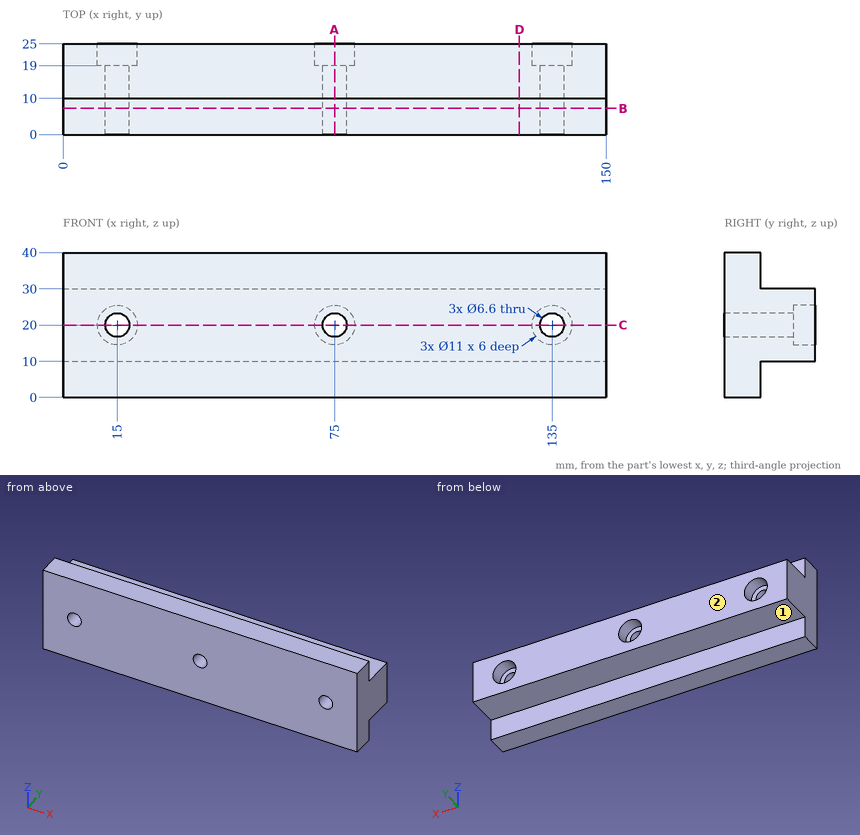
The drawing under review shows one solid part. Ordinate dimensions are in mm from its lowest x, y, z. A direction names the side the tool comes from. Round coordinates to 2 decimals unless told otherwise and drop trailing zeros. Loops run counter-clockwise (first coordinate to the right, second up) from the corner with the lowest first, then second, coordinate; pieces in that order, holes last.
Item 1: For the marked faces 1 and 2, list the 3-axis set-ups (+Z, -Z, +X, -X, +Y, -Y) from which the entire face can be reached by the end or side of a thin tool; tool diameter is ignored.
Determined:
face 1: -Z, +X, -X, +Y
face 2: +Z, -Z, +X, -X, +Y
Item 2: Take a section at A-A (x = 75). Write out the cut boundary in (y, z), then the cut area to 3 significant figures.
Determined:
outline: (0, 0) - (10, 0) - (10, 10) - (25, 10) - (25, 14.5) - (19, 14.5) - (19, 16.7) - (0, 16.7) - close; (0, 23.3) - (19, 23.3) - (19, 25.5) - (25, 25.5) - (25, 30) - (10, 30) - (10, 40) - (0, 40) - close
area: 509 mm2
Item 3: Take a section at D-D (x = 126). Write out the cut boundary in (y, z), then the cut area to 3 significant figures.
Determined:
outline: (0, 0) - (10, 0) - (10, 10) - (25, 10) - (25, 30) - (10, 30) - (10, 40) - (0, 40) - close
area: 700 mm2
Item 4: Take a section at B-B (y = 7.25). Write out the cut boundary in (x, z).
Determined:
outline: (0, 0) - (150, 0) - (150, 40) - (0, 40) - close; hole circle Ø6.6 at (15, 20); hole circle Ø6.6 at (75, 20); hole circle Ø6.6 at (135, 20)
Item 5: For line 1 (X direction, y = 5.5, z = 20); line 2 (X direction, y = 22.85, z = 20); line 3 (Z direction, x = 135, y = 20.4), list the stretches that pass through material, from the lowest coordinate up.
Determined:
line 1: x = 0 to 11.7, 18.3 to 71.7, 78.3 to 131.7, 138.3 to 150
line 2: x = 0 to 9.5, 20.5 to 69.5, 80.5 to 129.5, 140.5 to 150
line 3: z = 10 to 14.5, 25.5 to 30
Item 6: Clearance check with flat-ended pins moving along their axes: pin 1 Ø7.5 at (x, y) = (48.5, 18.5) entering from +Z; pin 2 Ø1 at (y, z) = (12, 34.5) entering from +X; pin 3 Ø3 at (x, z) = (88, 7.5) entering from +Y; pin 4 Ø4.5 at (x, y) = (74, 19) entering from -Z. State where each tip first meets the part, or that it passes through.
Determined:
pin 1: stops at z = 30
pin 2: passes through
pin 3: stops at y = 10
pin 4: stops at z = 10
Item 7: Take a section at C-C (z = 20). Write out the cut boundary in (x, y), then the cut area to 3 significant figures.
Determined:
outline: (0, 0) - (11.7, 0) - (11.7, 19) - (9.5, 19) - (9.5, 25) - (0, 25) - close; (18.3, 0) - (71.7, 0) - (71.7, 19) - (69.5, 19) - (69.5, 25) - (20.5, 25) - (20.5, 19) - (18.3, 19) - close; (78.3, 0) - (131.7, 0) - (131.7, 19) - (129.5, 19) - (129.5, 25) - (80.5, 25) - (80.5, 19) - (78.3, 19) - close; (138.3, 0) - (150, 0) - (150, 25) - (140.5, 25) - (140.5, 19) - (138.3, 19) - close
area: 3,180 mm2
